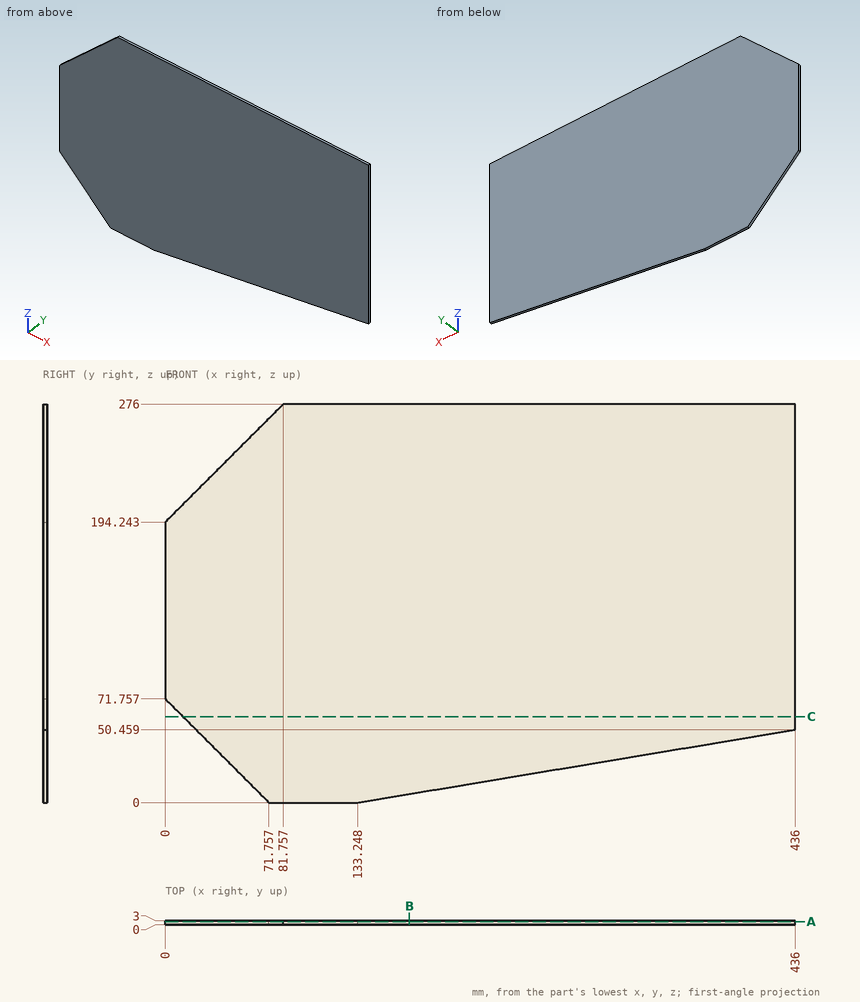
Print and shaded views of the part. All mm, measured from the part's lowest x, y and z. Round coordinates to 2 decimals unless told otherwise and drop trailing zeros. Write each loop counter-clockwise with the first axis right and the second up, starting at its lowest first coordinate (ties: lowest second). Pieces come first, ordered by that corner, then holes. Notation, with made-up numbers: M 13.5,-34.5 L 57.5,-34.5 A23 ccw 57.5,-18.5 Z; hole C 72,75.25 d8. An arc over 180 degrees is marked long. One line per question, with ' | ' between items.
(1) Probe line 1 along X through (y, z) = (1.7, 236.5); line 2 along X through (y, z) = (0.7, 262); line 3 along Z through (x, y) = (222, 2.35). List the from-to ranges inside material, lowest first.
Answer key:
line 1: x = 42.26 to 436 | line 2: x = 67.76 to 436 | line 3: z = 14.79 to 276
(2) Pin check, flat tip, straight feed: pin 1 (1.5 mm diameter, centred on y = 0.5, z = 38.5, fed in from -X). Stop position of the tip, or through.
Answer key:
pin 1: stops at x = 32.51
(3) Saw through at B-B on x = 169. Write the cut outline in (y, z).
Answer key:
outline: M 0,5.96 L 3,5.96 L 3,276 L 0,276 Z
(4) Saw through at C-C on z = 59.5. Write the cut outline in (x, y).
Answer key:
outline: M 12.26,0 L 436,0 L 436,3 L 12.26,3 Z
(5) Saw through at A-A on y = 2.25. Write the cut outline in (x, z), then the cut area to 3 significant figures.
Answer key:
outline: M 0,71.76 L 71.76,0 L 133.25,0 L 436,50.46 L 436,276 L 81.76,276 L 0,194.24 Z | area: 107,000 mm^2
